```python
from build123d import *

# Parameters (mm, degrees)
BASE_R              = 3.175
BOSS_EXTRUDE1_DEPTH = 12.7
ROUTER_FILLET_R     = 3.175


with BuildPart() as part:
    # base → Boss-Extrude1 (new body)
    with BuildSketch(Plane(origin=(0, 0, 0), x_dir=(1, 0, 0), z_dir=(0, 1, 0))):
        Polygon((0, 144.779530825), (38.1, 144.779530825), (59.224940876, 98.580214023), (190.5, 50.8), (190.5, 0), (0, 0), align=None)
        with Locations(Location((166.631807432, 51.378277014, 0), (0, 0, 270))):
            Circle(BASE_R, mode=Mode.SUBTRACT)
        with Locations(Location((36.451337699, 130.060960493, 0), (0, 0, 270))):
            Circle(BASE_R, mode=Mode.SUBTRACT)
        with Locations(Location((182.88, 45.464418559, 0), (0, 0, 270))):
            Circle(BASE_R, mode=Mode.SUBTRACT)
        with Locations(Location((68.552843668, 87.076100432, 0), (0, 0, 270))):
            Circle(BASE_R, mode=Mode.SUBTRACT)
        with Locations(Location((47.013808137, 106.961302092, 0), (0, 0, 270))):
            Circle(BASE_R, mode=Mode.SUBTRACT)
        with Locations(Location((182.88, 7.62, 0), (0, 0, 270))):
            Circle(BASE_R, mode=Mode.SUBTRACT)
        with Locations(Location((7.62, 7.62, 0), (0, 0, 270))):
            Circle(BASE_R, mode=Mode.SUBTRACT)
        with Locations(Location((7.62, 106.679530825, 0), (0, 0, 270))):
            Circle(BASE_R, mode=Mode.SUBTRACT)
        with Locations(Location((25.4, 7.62, 0), (0, 0, 270))):
            Circle(BASE_R, mode=Mode.SUBTRACT)
        with Locations(Location((165.1, 7.62, 0), (0, 0, 270))):
            Circle(BASE_R, mode=Mode.SUBTRACT)
        with Locations(Location((25.4, 25.4, 0), (0, 0, 270))):
            Circle(BASE_R, mode=Mode.SUBTRACT)
        with Locations(Location((114.3, 25.4, 0), (0, 0, 270))):
            Circle(BASE_R, mode=Mode.SUBTRACT)
        with BuildLine():
            Line((95.25, 12.7), (44.45, 12.7))
            ThreePointArc((44.45, 12.7), (31.75, 25.4), (44.45, 38.1))
            Line((44.45, 38.1), (95.25, 38.1))
            ThreePointArc((95.25, 38.1), (107.95, 25.4), (95.25, 12.7))
        make_face(mode=Mode.SUBTRACT)
    extrude(amount=BOSS_EXTRUDE1_DEPTH)

    # router_fillet
    router_fillet_edges = [part.edges().sort_by_distance(p)[0] for p in [
        (0, 6.35, -144.779530825),
        (38.1, 6.35, -144.779530825),
        (59.224940876, 6.35, -98.580214023),
        (190.5, 6.35, -50.8),
        (190.5, 6.35, 0),
        (0, 6.35, 0),
    ]]
    fillet(router_fillet_edges, radius=ROUTER_FILLET_R)


solid = part.part
```
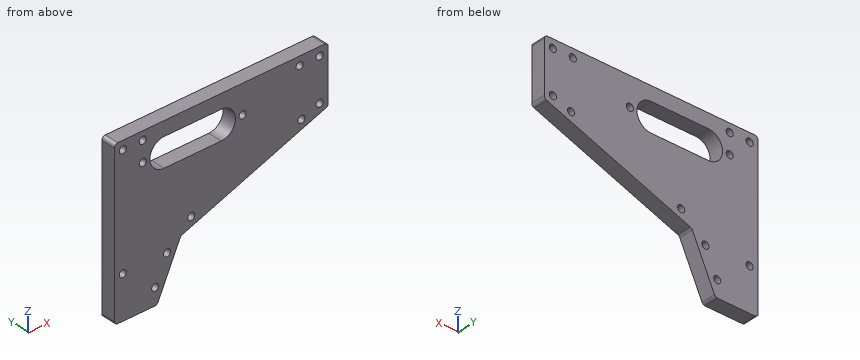
The model under review builds one solid part; all positions refer to its coordinate system, in mm. Give positions to 0.01 mm unless a question says otherwise; leave off trailing zeros. Write each loop counter-clockwise with the first axis right and the second up, starting at its lowest first coordinate (ties: lowest second). Pieces come first, ordered by that corner, then holes.
(1) For P1, Ø10, axis at x = 25.4, z = -7.62, coming from the +Y side; P2, Ø1, axis at x = 70, y = 8.5, coming from the -Z side; P3, Ø6.5, axis at x = 68.5, y = 6, coming from the -Z side, all flat-tipped, find the tip position at first contact; note any pin that passes through.
(2) Consider section C-C, the plane x = 114.3. Give the boundary of the cut face in (y, z) (3 decimals), and give its area (3 significant figures).
(3) Consider section B-B, the plane x = 25.4. Give the boundary of the cut face in (y, z) (3 decimals), and give its area (3 significant figures).
(4) To check wall thickness, follow L1, parallel to X at y = 9.25, z = -7.62 (3 decimals); L2, parallel to X at y = 9.5, z = -25.4 (3 decimals); L3, parallel to X at y = 4.25, z = -27. State the ranges of each line that lie inside material, in increasing order.
(5) Consider section A-A, the plane z = -7.62. Give the boundary of the cut face in (x, y) (3 decimals), and give its area (3 significant figures).
(6) Consider section D-D, the plane z = -107. Give the boundary of the cut face in (x, y), and give its area (3 significant figures).
Returned:
1. P1: stops at y = 12.7
1. P2: stops at z = -94.84
1. P3: stops at z = -96.39
2. outline: (0, -78.535) - (12.7, -78.535) - (12.7, -28.575) - (0, -28.575) - close; (0, -22.225) - (12.7, -22.225) - (12.7, 0) - (0, 0) - close
2. area: 917 mm2
3. outline: (0, -144.78) - (12.7, -144.78) - (12.7, -28.575) - (0, -28.575) - close; (0, -22.225) - (12.7, -22.225) - (12.7, -10.795) - (0, -10.795) - close; (0, -4.445) - (12.7, -4.445) - (12.7, 0) - (0, 0) - close
3. area: 1,680 mm2
4. L1: x = 0 to 4.445, 10.795 to 22.225, 28.575 to 161.925, 168.275 to 179.705, 186.055 to 190.5
4. L2: x = 0 to 22.225, 28.575 to 31.75, 107.95 to 111.125, 117.475 to 190.5
4. L3: x = 0 to 22.66, 28.14 to 31.85, 107.85 to 111.56, 117.04 to 190.5
5. outline: (0, 0) - (4.445, 0) - (4.445, 12.7) - (0, 12.7) - close; (10.795, 0) - (22.225, 0) - (22.225, 12.7) - (10.795, 12.7) - close; (28.575, 0) - (161.925, 0) - (161.925, 12.7) - (28.575, 12.7) - close; (168.275, 0) - (179.705, 0) - (179.705, 12.7) - (168.275, 12.7) - close; (186.055, 0) - (190.5, 0) - (190.5, 12.7) - (186.055, 12.7) - close
5. area: 2,100 mm2
6. outline: (0, 0) - (4.46, 0) - (4.46, 12.7) - (0, 12.7) - close; (10.78, 0) - (43.84, 0) - (43.84, 12.7) - (10.78, 12.7) - close; (50.19, 0) - (55.37, 0) - (55.37, 12.7) - (50.19, 12.7) - close
6. area: 542 mm2
